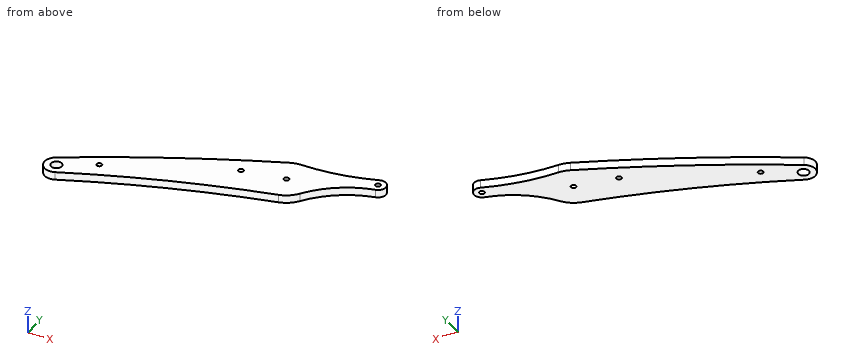
from build123d import *

# Parameters (mm, degrees)
SKETCH1_R           = 1.95
SKETCH1_R_2         = 4.1
BOSS_EXTRUDE1_DEPTH = 6


with BuildPart() as part:
    # Sketch1 → Boss-Extrude1 (new body)
    with BuildSketch(Plane.XY):
        with BuildLine():
            ThreePointArc((-249.547735749, 127.673100022), (-252.877471407, 115.79000474), (-241.215192405, 111.754370772))
            ThreePointArc((-241.215192405, 111.754370772), (-170.350070338, 139.847528819), (-97.252990361, 161.478708942))
            ThreePointArc((-97.252990361, 161.478708942), (-90.570551573, 164.523097822), (-85.437324527, 169.774123618))
            ThreePointArc((-85.437324527, 169.774123618), (-67.229564843, 188.321481613), (-43.509998386, 198.94735421))
            ThreePointArc((-43.509998386, 198.94735421), (-39.165402052, 206.535635416), (-47.008101374, 210.402106199))
            ThreePointArc((-47.008101374, 210.402106199), (-73.946915163, 203.086860773), (-101.774691803, 200.889737355))
            ThreePointArc((-101.774691803, 200.889737355), (-105.950118059, 200.510334794), (-109.954702491, 199.268789688))
            ThreePointArc((-109.954702491, 199.268789688), (-180.973525069, 165.854124566), (-249.547735749, 127.673100022))
        make_face()
        with Locations((-102.0625187, 180.89180857)):
            Circle(SKETCH1_R, mode=Mode.SUBTRACT)
        with Locations((-44.903785826, 204.783222318)):
            Circle(SKETCH1_R, mode=Mode.SUBTRACT)
        with Locations((-244.903785826, 119.963772612)):
            Circle(SKETCH1_R_2, mode=Mode.SUBTRACT)
        with Locations((-219.903785826, 134.304249979)):
            Circle(SKETCH1_R, mode=Mode.SUBTRACT)
        with Locations((-133.8125187, 175.069049716)):
            Circle(SKETCH1_R, mode=Mode.SUBTRACT)
    extrude(amount=BOSS_EXTRUDE1_DEPTH)


solid = part.part
Model file for the job. Use its own axes, mm. Give positions to 0.01 mm unless a question says otherwise; leave off trailing zeros. Write each loop counter-clockwise with the first axis right and the second up, starting at its lowest first coordinate (ties: lowest second). Pieces come first, ordered by that corner, then holes. Notation, with made-up numbers: (12.5, 50) -> (42.5, 50) arc R6 ccw to (42.5, 54) -> close; hole circle Ø8 at (-6.75, 27). An arc over 180 degrees is marked (long way). Write item = value, one per line.
(1) Slice it at A-A, the plane y = 122. Give the cut face in (x, z), then the cut area to 3 significant figures.
Determined:
outline = (-253.67, 0) -> (-248.46, 0) -> (-248.46, 6) -> (-253.67, 6) -> close; (-241.35, 0) -> (-217.45, 0) -> (-217.45, 6) -> (-241.35, 6) -> close
area = 175 mm2
(2) Slice it at D-D, the plane y = 186. Give the cut face in (x, z), then the cut area to 3 significant figures.
Determined:
outline = (-139.68, 0) -> (-70.37, 0) -> (-70.37, 6) -> (-139.68, 6) -> close
area = 416 mm2
(3) Slice it at B-B, the plane z = 4.6. Give the cut face in (x, y).
Determined:
outline = (-249.55, 127.67) arc R9 ccw to (-241.22, 111.75) arc R850 cw to (-97.25, 161.48) arc R20 ccw to (-85.44, 169.77) arc R70 cw to (-43.51, 198.95) arc R6 ccw (long way) to (-47.01, 210.4) arc R150 cw to (-101.77, 200.89) arc R20 ccw to (-109.95, 199.27) arc R1150 ccw to start; hole circle Ø8.2 at (-244.9, 119.96); hole circle Ø3.9 at (-219.9, 134.3); hole circle Ø3.9 at (-133.81, 175.07); hole circle Ø3.9 at (-102.06, 180.89); hole circle Ø3.9 at (-44.9, 204.78)
(4) Slice it at C-C, the plane x = -193. Give the cut face in (y, z), then the cut area to 3 significant figures.
Determined:
outline = (131.66, 0) -> (159.6, 0) -> (159.6, 6) -> (131.66, 6) -> close
area = 168 mm2
(5) Probe line 1 along X through (y, z) = (180.5, 1.45); line 2 along Y through (x, z) = (-243.5, 2.35); line 3 along X through (y, z) = (122.5, 1.05). List the from-to ranges inside material, lowest first.
Determined:
line_1 = -151.38 to -103.97, -100.15 to -76.61
line_2 = 111.07 to 116.11, 123.82 to 131.29
line_3 = -253.54 to -248.13, -241.68 to -216.24
(6) Flat gauge pins, fed straight in: P1, Ø13, axis at x = -244.9, y = 119.96, coming from the +Z side; P2, Ø1.5, axis at y = 164, z = 3.5, coming from the -X side; P3, Ø1, axis at x = -138.5, z = 2.5, coming from the -Y side. Where does each tip first touch, or does it go through?
Determined:
P1 = 6
P2 = -186.02
P3 = 150
